from build123d import *

# Parameters (mm, degrees)
ESBO_O1_R                = 2.1
ESBO_O1_R_2              = 2
ESBO_O1_R_3              = 12
RESSALTO_EXTRUS_O1_DEPTH = 10
RESSALTO_EXTRUS_O2_DEPTH = 17.2
ESBO_O3_R                = 1.2
CORTE_EXTRUS_O1_DEPTH    = 3
NERVURA1_REACH           = 155.293
ESBO_O4_WALL_W           = 333.586365546
ESBO_O4_WALL_H           = 2.5
ESBO_O5_R                = 2.025
CORTE_EXTRUS_O2_DEPTH    = 1.5


with BuildPart() as part:
    # Esboço1 → Ressalto-extrusão1 (new body)
    with BuildSketch(Plane.XY):
        with BuildLine():
            Line((-51.961524227, -65), (51.961524227, -65))
            ThreePointArc((51.961524227, -65), (82.27241336, -47.5), (82.27241336, -12.5))
            Line((82.27241336, -12.5), (30.310889132, 77.5))
            ThreePointArc((30.310889132, 77.5), (0, 95), (-30.310889132, 77.5))
            Line((-30.310889132, 77.5), (-82.27241336, -12.5))
            ThreePointArc((-82.27241336, -12.5), (-82.27241336, -47.5), (-51.961524227, -65))
        make_face()
        with Locations((-12, 70)):
            Circle(ESBO_O1_R, mode=Mode.SUBTRACT)
        with Locations((-66.621778265, -24.607695155)):
            Circle(ESBO_O1_R, mode=Mode.SUBTRACT)
        with Locations(Location((12, 70, 0), (0, 0, 180))):
            Circle(ESBO_O1_R, mode=Mode.SUBTRACT)
        with Locations(Location((-54.621778265, -45.392304845, 0), (0, 0, 180))):
            Circle(ESBO_O1_R, mode=Mode.SUBTRACT)
        with Locations((66.621778265, -24.607695155)):
            Circle(ESBO_O1_R, mode=Mode.SUBTRACT)
        with Locations((54.621778265, -45.392304845)):
            Circle(ESBO_O1_R, mode=Mode.SUBTRACT)
        with Locations((31.83350832, -36.842746207)):
            Circle(ESBO_O1_R_2, mode=Mode.SUBTRACT)
        with Locations((25.980762114, -15)):
            Circle(ESBO_O1_R_3, mode=Mode.SUBTRACT)
        with Locations((4.138015907, -20.852746207)):
            Circle(ESBO_O1_R_2, mode=Mode.SUBTRACT)
        with Locations((20.128015907, 6.842746207)):
            Circle(ESBO_O1_R_2, mode=Mode.SUBTRACT)
        with Locations((47.82350832, -9.147253793)):
            Circle(ESBO_O1_R_2, mode=Mode.SUBTRACT)
    extrude(amount=RESSALTO_EXTRUS_O1_DEPTH)

    # Esboço2 → Ressalto-extrusão2 (add)
    with BuildSketch(Plane.XY.offset(10)):
        Polygon((-36.821647177, 21.223079253), (-15.188309322, 8.693167311), (-13.684719889, 11.289167854), (-35.318057744, 23.819079795), align=None)
    extrude(amount=RESSALTO_EXTRUS_O2_DEPTH)

    # Esboço3 → Corte-extrusão1 (cut)
    with BuildSketch(Plane(origin=(-0.045026547, -0.077739931, 0), x_dir=(0.8653335141925842, -0.5011964776563306, 0), z_dir=(-0.5011964776563306, -0.8653335141925842, 0))):
        with Locations((-34.749937916, 19.5)):
            Circle(ESBO_O3_R)
        with Locations((-25.249937916, 19.5)):
            Circle(ESBO_O3_R)
    extrude(amount=-CORTE_EXTRUS_O1_DEPTH, mode=Mode.SUBTRACT)

    # Esboço4 wall → Nervura1 (add, up to next)
    with BuildSketch(Plane(origin=(-39.954125162, 15.814744789, 16.374682453), x_dir=(-0.250598238796, -0.432666757113, -0.866025403786), z_dir=(-0.434048881938, -0.749400806038, 0.499999999998)), mode=Mode.PRIVATE) as nervura1_sk1:
        with Locations((0, 1.25)):
            Rectangle(ESBO_O4_WALL_W, ESBO_O4_WALL_H)
    nervura1_tool1 = extrude(nervura1_sk1.sketch, amount=-NERVURA1_REACH, mode=Mode.PRIVATE) - part.part
    nervura1 = nervura1_tool1.solids().sort_by_distance((-39.954125162, 15.814744789, 16.374682453))[0]
    add(nervura1)

    # Espelhar1: Nervura1 across plane
    add(nervura1.mirror(Plane(origin=(-25.959951703, 15.035863214, 0), x_dir=(0, 0, 1), z_dir=(-0.8653335141925849, 0.5011964776563297, 0))))

    # Esboço5 → Corte-extrusão2 (cut)
    with BuildSketch(Plane.XY.offset(10)):
        with Locations((-78.808311744, -14.5)):
            Circle(ESBO_O5_R)
        with Locations((-51.961524227, -61)):
            Circle(ESBO_O5_R)
        with Locations((26.846787517, 75.5)):
            Circle(ESBO_O5_R)
        with Locations((44.166787517, 45.500880013)):
            Circle(ESBO_O5_R)
        with Locations((61.486787517, 15.501760026)):
            Circle(ESBO_O5_R)
        with Locations((78.806787517, -14.497359961)):
            Circle(ESBO_O5_R)
        with Locations((-61.488311744, 15.499119987)):
            Circle(ESBO_O5_R)
        with Locations((-44.168311744, 45.498239974)):
            Circle(ESBO_O5_R)
        with Locations((-26.848311744, 75.497359961)):
            Circle(ESBO_O5_R)
        with Locations((-17.321524227, -61)):
            Circle(ESBO_O5_R)
        with Locations((17.318475773, -61)):
            Circle(ESBO_O5_R)
        with Locations((51.958475773, -61)):
            Circle(ESBO_O5_R)
    extrude(amount=-CORTE_EXTRUS_O2_DEPTH, mode=Mode.SUBTRACT)


solid = part.part
Model file for the job. Use its own axes, mm. A direction names the side the tool comes from. Give positions to 0.01 mm unless a question says otherwise; leave off trailing zeros. Order: outer loops, then holes, each group sorted by start corner. A loop starts at its lowest first (then second) coordinate and runs counter-clockwise, first axis right, second up. Notation, with made-up numbers: (-13, 0.25) -> (3, 0.25) arc R25 ccw to (3, 20.25) -> close; hole circle Ø2 at (69, 65.25). An arc over 180 degrees is marked (long way). Use CSV: the item, a comma, the result in double quotes.
1. Band-saw the part on D-D, the plane y = 64. Give the cut face in (x, z).
Outcome:
outline,"(-38.11, 0) -> (38.11, 0) -> (38.11, 10) -> (-38.11, 10) -> close"
2. Mould opens along X. For faces 3 (the flat face through (-25, 16, 27.2)), 4 (the cylindrical face through (-80.83, -14.41, 9.26)), 5 (the cylindrical face through (-52.401, -62.977, 9.26)), 6 (the flat face through (-24.35, 17.466, 18.48)) say: +X half, -X half, draft (parallel to the pull), parting line (faces both ways), or undercut.
Outcome:
face 3,"draft"
face 4,"undercut"
face 5,"undercut"
face 6,"+X half"
3. 3-axis set-ups, long thin cutter, end or side, ignore diameter. For faces 1 (the cylindrical face through (64.524, -24.515, 4.93)), 2 (the flat face through (-62, 16, 8.5)): which of +Z, -Z, +X, -X, +Y, -Y reach the whole face in a straight line?
Outcome:
face 1,"+Z, -Z"
face 2,"+Z"
4. Band-saw the part on A-A, the plane x = 12. Give the cut face in (y, z), then the cut area to 3 significant figures.
Outcome:
outline,"(-65, 0) -> (67.9, 0) -> (67.9, 10) -> (-65, 10) -> close; (72.1, 0) -> (92.88, 0) -> (92.88, 10) -> (72.1, 10) -> close"
area,"1,540 mm²"
5. Drill centre lines: line 1 along Z through (x, y) = (78, -27.5); line 2 along Y through (x, z) = (3.5, 8.25); line 3 along X through (y, z) = (-10.5, 3.5). Where is each one in solid material? Low to high. Write a range as from..to.
Outcome:
line 1,"0..10"
line 2,"-65..-22.75, -18.96..94.82"
line 3,"-81.12..14.86, 37.11..46.35, 49.3..81.12"
6. Drop flat-ended pins along their axis: pin 1 (1.2 mm diameter, centred on x = -52, y = -61.5, fed in from +Z); pin 2 (6 mm diameter, centred on x = -27, z = 11.5, fed in from +Y); pin 3 (4.5 mm diameter, centred on x = 52, y = -62, fed in from +Z); pin 4 (4 mm diameter, centred on x = -66.62, y = -24.61, fed in from +Z). Give the stop position or say it passes through.
Outcome:
pin 1,"z = 8.5"
pin 2,"y = 85.09"
pin 3,"z = 10"
pin 4,"through"
7. Band-saw the part on B-B, the plane y = -61. Give the cut face in (x, z), then the cut area to 3 significant figures.
Outcome:
outline,"(-68.21, 0) -> (68.21, 0) -> (68.21, 10) -> (53.98, 10) -> (53.98, 8.5) -> (49.93, 8.5) -> (49.93, 10) -> (19.34, 10) -> (19.34, 8.5) -> (15.29, 8.5) -> (15.29, 10) -> (-15.3, 10) -> (-15.3, 8.5) -> (-19.35, 8.5) -> (-19.35, 10) -> (-49.94, 10) -> (-49.94, 8.5) -> (-53.99, 8.5) -> (-53.99, 10) -> (-68.21, 10) -> close"
area,"1,340 mm²"
8. Band-saw the part on C-C, the plane z = 24. Give the cut face in (x, y), then the cut area to 3 significant figures.
Outcome:
outline,"(-37.75, 19.62) -> (-35.58, 18.37) -> (-34.66, 19.97) -> (-17.35, 9.95) -> (-18.28, 8.35) -> (-16.11, 7.09) -> (-13.68, 11.29) -> (-35.32, 23.82) -> close"
area,"84.2 mm²"
